For this review, take the finished solid that the model builds, in its own axes (mm). A direction names the side the tool comes from. Give positions to 0.01 mm unless a question says otherwise; leave off trailing zeros. Use one line per item in the form item = value. Start each with the question number.
Q1. Consider section A-A on x = 0. Give the number of separate pieces and of enclosed holes in the cut face, and give its area (3 significant figures).
Q2. Clearance check with flat-ended pins moving along their axes: pin 1 Ø1.5 at (y, z) = (-11, -9) entering from +X; pin 2 Ø6 at (x, z) = (-2, -7.5) entering from -Y; pin 3 Ø3 at (x, z) = (-7, 0) entering from -Y; pin 4 Ø1 at (x, y) = (-3, -11.5) entering from -Z. State where each tip first meets the part, or that it passes through.
Q3. For probe 1 along Z at (x, y) = (0, -4.5); probe 2 along X at (y, z) = (-2.5, -1.25); probe 3 along X at (y, z) = (-4.75, -1), list the stretches that pass through material, from the lowest coordinate up. Write a range as [from, to].
Q4. Mouldability with a two-part tool opening along Z and no side actions: class faces 4 (the cylindrical face through (0.831, -3.457, -8.597)), 5 (the cylindrical face through (-2.05, -3.41, 7.46)), 6 (the conical face through (0.51, -6.89, -14.7)) as released by +Z, released by -Z, zero draft, split by the parting line, or undercut.
Q5. Tool access review of faces 1 (the conical face through (0.52, -3.34, -14.15)), 2 (the flat face through (7.17, -9.72, -5.05)), 3 (the flat face through (-7.17, -9.72, 5.05)): name each direction out of +Z, -Z, +X, -X, +Y, -Y from which nothing blocks a thin tool from reaching the whole face with its end or side.
```python
from build123d import *

# Parameters (mm, degrees)
SKETCH017_R        = 15
SKETCH017_R_2      = 4
SKETCH017_R_3      = 1.8
PAD005_DEPTH       = 7
SKETCH020_W        = 18
SKETCH020_H        = 3
POCKET010_DEPTH    = 7.001
SKETCH021_R        = 2.05
POCKET011_DEPTH    = 12.001
CHAMFER009_SIZE    = 0.4
PAD023_DEPTH       = 1.5
POLARPATTERN_COUNT = 2
FILLET020_R        = 3
CHAMFER037_SIZE    = 0.4


with BuildPart() as part:
    # Sketch017 → Pad005 (new body)
    with BuildSketch(Plane.XZ):
        Circle(SKETCH017_R)
        Circle(SKETCH017_R_2, mode=Mode.SUBTRACT)
        with Locations((-7, 0)):
            Circle(SKETCH017_R_3, mode=Mode.SUBTRACT)
        with Locations((0, -7)):
            Circle(SKETCH017_R_3, mode=Mode.SUBTRACT)
        with Locations((7, 0)):
            Circle(SKETCH017_R_3, mode=Mode.SUBTRACT)
    extrude(amount=PAD005_DEPTH)

    # Sketch018 → Groove (revolve, cut)
    with BuildSketch(Plane.XY):
        Polygon((15, -2.5), (14, -3.5), (15, -4.5), align=None)
    revolve(axis=Axis((0, 0, 0), (0, 1, 0)), mode=Mode.SUBTRACT)

    # Sketch020 → Pocket010 (cut, through all)
    with BuildSketch(Plane.XZ):
        with Locations((0, 13.5)):
            Rectangle(SKETCH020_W, SKETCH020_H)
    extrude(amount=POCKET010_DEPTH, mode=Mode.SUBTRACT)

    # Sketch021 → Pocket011 (cut, through all)
    with BuildSketch(Plane.XY):
        with Locations((0, -3.5)):
            Circle(SKETCH021_R)
    extrude(amount=POCKET011_DEPTH, mode=Mode.SUBTRACT)

    # Chamfer009
    chamfer009_edges = [part.edges().sort_by_distance(p)[0] for p in [
        (-2.05, -3.5, 12),
        (13.416408, 0, 6.708204),
        (0, 0, 12),
        (-6.708204, 0, -13.416408),
        (-8.8, 0, 0),
        (-1.8, 0, -7),
        (-4, 0, 0),
        (5.2, 0, 0),
        (13.416408, -7, 6.708204),
        (0, -7, 12),
        (-6.708204, -7, -13.416408),
        (-8.8, -7, 0),
        (-1.8, -7, -7),
        (-4, -7, 0),
        (5.2, -7, 0),
    ]]
    chamfer(chamfer009_edges, length=CHAMFER009_SIZE)

    # Sketch055 (on Plane of DatumPlane001) → Pad023 (join, symmetric)
    with BuildSketch(Plane(origin=(0, 0, 0), x_dir=(0.707107, 0, -0.707107), z_dir=(0.707107, 0, 0.707107))):
        with BuildLine():
            ThreePointArc((-14, -7), (-11.124423, -12.964434), (-5.874887, -17))
            Line((-5, -7), (-5.874887, -17))
            Line((-14, -7), (-5, -7))
        make_face()
    pad023 = extrude(amount=PAD023_DEPTH, both=True)

    # PolarPattern: Pad023 ×2 about axis
    polarpattern_axis = Axis((0, 0, 0), (0, 1, 0))
    for i in range(1, POLARPATTERN_COUNT):
        add(pad023.rotate(polarpattern_axis, i * 360 / POLARPATTERN_COUNT))

    # Fillet020
    fillet020_edges = [part.edges().sort_by_distance(p)[0] for p in [
        (-4.154172, -17, 4.154172),
        (4.154172, -17, -4.154172),
    ]]
    fillet(fillet020_edges, radius=FILLET020_R)

    # Chamfer037
    chamfer037_edges = [part.edges().sort_by_distance(p)[0] for p in [
        (2.62296, -9.39375, -4.744281),
        (4.744281, -9.39375, -2.62296),
        (-4.744281, -9.39375, 2.62296),
        (-2.62296, -9.39375, 4.744281),
    ]]
    chamfer(chamfer037_edges, length=CHAMFER037_SIZE)


solid = part.part
```
Working result:
q1.separate_pieces = 4
q1.enclosed_holes = 0
q1.area = 72.9 mm²
q2.pin_1 = 9.58
q2.pin_2 = -7
q2.pin_3 = through
q2.pin_4 = 4.12
q3.probe_1 = [-15, -8.8], [-5.2, -4]
q3.probe_2 = [-14.95, -8.3], [-5.7, -3.8], [3.8, 5.7], [8.3, 14.95]
q3.probe_3 = [-14.97, -8.5], [-5.5, -3.87], [3.87, 5.5], [8.5, 14.97]
q4.face_4 = undercut
q4.face_5 = zero draft
q4.face_6 = split by the parting line
q5.face_1 = none
q5.face_2 = +Z, +X, -Y
q5.face_3 = -Z, -X, -Y
